Verification items for this drawing (mm, ordinates from the low corner). Coordinates: 2 decimals unless noted, no trailing zeros. Write each loop counter-clockwise with the first axis right and the second up, starting at its lowest first coordinate (ties: lowest second). Pieces come first, ordered by that corner, then holes. Notation, with made-up numbers: (35.5, 83) -> (40.5, 83) arc R22 ccw to (40.5, 94) -> close; hole circle Ø6 at (25, -29.5). An arc over 180 degrees is marked (long way). Use CSV: the item, a comma, the result in double quotes.
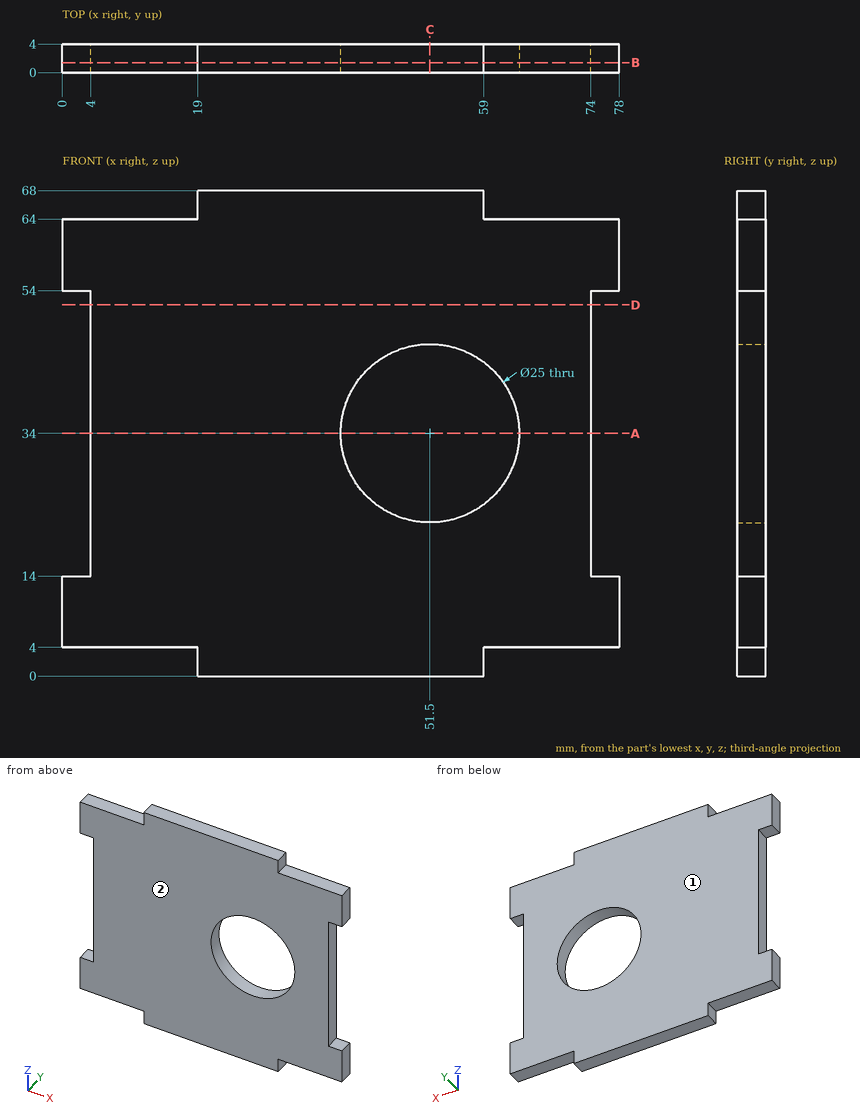
1) Cross-section at D-D (z = 52). Record the boundary of the cut face in (x, y), plus the area to 3 significant figures.
Return value:
outline,"(4, 0) -> (74, 0) -> (74, 4) -> (4, 4) -> close"
area,"280 mm2"
2) Cross-section at B-B (y = 1.4). Record the boundary of the cut face in (x, z).
Return value:
outline,"(0, 4) -> (19, 4) -> (19, 0) -> (59, 0) -> (59, 4) -> (78, 4) -> (78, 14) -> (74, 14) -> (74, 54) -> (78, 54) -> (78, 64) -> (59, 64) -> (59, 68) -> (19, 68) -> (19, 64) -> (0, 64) -> (0, 54) -> (4, 54) -> (4, 14) -> (0, 14) -> close; hole circle Ø25 at (51.5, 34)"
3) Mould release check, pull along Y, two halves, no side actions. Record for the marked faces 1 and 2: released by +Y, released by -Y, zero draft, split by the parting line, or undercut.
Return value:
face 1,"released by +Y"
face 2,"released by -Y"
4) Cross-section at C-C (x = 51.5). Record the boundary of the cut face in (y, z), plus the area to 3 significant figures.
Return value:
outline,"(0, 0) -> (4, 0) -> (4, 21.5) -> (0, 21.5) -> close; (0, 46.5) -> (4, 46.5) -> (4, 68) -> (0, 68) -> close"
area,"172 mm2"
5) Scan lines: L1, parallel to X at y = 2, z = 34; L2, parallel to Z at x = 51.5, y = 0.9; L3, parallel to X at y = 3.4, z = 65.5. Record each from-to range of solid material in increasing order.
Return value:
L1,"4 to 39, 64 to 74"
L2,"0 to 21.5, 46.5 to 68"
L3,"19 to 59"
6) Cross-section at A-A (z = 34). Record the boundary of the cut face in (x, y).
Return value:
outline,"(4, 0) -> (39, 0) -> (39, 4) -> (4, 4) -> close; (64, 0) -> (74, 0) -> (74, 4) -> (64, 4) -> close"
7) Gauge pin test, flat ends, axial feed: pin 1 (1.2 mm diameter, centred on x = 75, y = 2.5, fed in from -Z); pin 2 (1.2 mm diameter, centred on y = 2, z = 66.5, fed in from -X); pin 3 (2 mm diameter, centred on y = 2, z = 2.5, fed in from +X). Record the tip position at first contact, or that the pin passes through.
Return value:
pin 1,"z = 4"
pin 2,"x = 19"
pin 3,"x = 59"
